from build123d import *

# Parameters (mm, degrees)
SKETCH1_W                              = 60
SKETCH1_H                              = 60
BOSS_EXTRUDE1_DEPTH                    = 3
SKETCH2_R                              = 10.25
CUT_EXTRUDE1_DEPTH                     = 43.532340636
SKETCH3_R                              = 1.45
SERVO_Y_MOUNT_D2P9_DEPTH               = 3.01
SKETCH4_R                              = 1.45
CUT_EXTRUDE5_DEPTH                     = 43.532340636
SKETCH5_R                              = 1.2
GUIDERAIL1_D2P4_DEPTH                  = 3.01
SKETCH6_R                              = 1.2
GUIDEBLOCK2_D2P4_DEPTH                 = 3.01
SKETCH7_R                              = 2.1
GUIDEBLOCK2_HEADCOUNTERBORE_D4P2_DEPTH = 2.05


with BuildPart() as part:
    # Sketch1 → Boss-Extrude1 (new body)
    with BuildSketch(Plane.XY):
        Rectangle(SKETCH1_W, SKETCH1_H)
    extrude(amount=BOSS_EXTRUDE1_DEPTH)

    # Sketch2 → Cut-Extrude1 (cut, through all)
    with BuildSketch(Plane.XY.offset(3)):
        Circle(SKETCH2_R)
    extrude(amount=-CUT_EXTRUDE1_DEPTH, mode=Mode.SUBTRACT)

    # Sketch3 → Servo_Y_Mount_D2p9 (cut)
    with BuildSketch(Plane(origin=(0, 0, 0), x_dir=(-1, 0, 0), z_dir=(0, 0, -1))):
        with Locations((18, -25)):
            Circle(SKETCH3_R)
        with Locations((25, -25)):
            Circle(SKETCH3_R)
    extrude(amount=-SERVO_Y_MOUNT_D2P9_DEPTH, mode=Mode.SUBTRACT)

    # Sketch4 → Cut-Extrude5 (cut, through all)
    with BuildSketch(Plane(origin=(0, 0, 0), x_dir=(-1, 0, 0), z_dir=(0, 0, -1))):
        with Locations((17, 27)):
            Circle(SKETCH4_R)
        with Locations((23, 27)):
            Circle(SKETCH4_R)
    extrude(amount=-CUT_EXTRUDE5_DEPTH, mode=Mode.SUBTRACT)

    # Sketch5 → GuideRail1_D2p4 (cut)
    with BuildSketch(Plane.XY.offset(3)):
        with Locations((-24, -15)):
            Circle(SKETCH5_R)
        with Locations((-24, 0)):
            Circle(SKETCH5_R)
        with Locations((-24, 15)):
            Circle(SKETCH5_R)
    extrude(amount=-GUIDERAIL1_D2P4_DEPTH, mode=Mode.SUBTRACT)

    # Sketch6 → GuideBlock2_D2p4 (cut)
    with BuildSketch(Plane.XY.offset(3)):
        with Locations((0, -28)):
            Circle(SKETCH6_R)
        with Locations((0, -20)):
            Circle(SKETCH6_R)
    extrude(amount=-GUIDEBLOCK2_D2P4_DEPTH, mode=Mode.SUBTRACT)

    # Sketch7 → GuideBlock2_HeadCounterbore_D4p2 (cut)
    with BuildSketch(Plane.XY.offset(3)):
        with Locations((0, -28)):
            Circle(SKETCH7_R)
        with Locations((0, -20)):
            Circle(SKETCH7_R)
    extrude(amount=-GUIDEBLOCK2_HEADCOUNTERBORE_D4P2_DEPTH, mode=Mode.SUBTRACT)


solid = part.part
Geometry: final body of the model. Coordinates: model frame, mm. A direction names the side the tool comes from. Give positions to 0.01 mm unless a question says otherwise; leave off trailing zeros. Order: outer loops, then holes, each group sorted by start corner. A loop starts at its lowest first (then second) coordinate and runs counter-clockwise, first axis right, second up. Notation, with made-up numbers: (-5, -22.5) - (15, -22.5) arc R30 cw to (15, 7.5) - close; hole circle Ø1 at (-6, 20). An arc over 180 degrees is marked (long way). Use CSV: the item, a comma, the result in double quotes.
1. Section query C-C (x = -7.5). Output: boundary loops of the cut face in (y, z), plus the area to 3 significant figures.
Answers below:
outline,"(-30, 0) - (-6.99, 0) - (-6.99, 3) - (-30, 3) - close; (6.99, 0) - (30, 0) - (30, 3) - (6.99, 3) - close"
area,"138 mm2"
2. Mould query, pull axis Y, two halves, no side actions, for faces 1 (the face through (30, 0, 1)), 2 (the face through (-0.4, -30, 0.8)), 3 (the face through (-19.339, -25.555, 1.479)). Classes: +Y half, -Y half, draft (parallel to the pull), parting line (faces both ways), or undercut.
Answers below:
face 1,"draft"
face 2,"-Y half"
face 3,"undercut"
3. Access query for faces 4 (the face through (1, -29, 0.95)), 5 (the face through (-25.2, 0.05, 1.52)). Directions: +Z, -Z, +X, -X, +Y, -Y. A direction counts if a zero-diameter tool reaches every point of the face in a straight line with its end or side. Return the directions, or none.
Answers below:
face 4,"+Z"
face 5,"+Z, -Z"
4. Contact query for a flat-ended pin moving along its axis: pin 1 (1.3 mm diameter, centred on x = 0.5, y = -21, fed in from +Z). Output: stop coordinate, or through.
Answers below:
pin 1,"z = 0.95"
5. Material intervals for line 1 along Y through (x, z) = (0, 2.3); line 2 along Y through (x, z) = (0, 0.4); line 3 along Y through (x, z) = (-24, 0.7), sorted ascending. Write a range as from..to.
Answers below:
line 1,"-25.9..-22.1, -17.9..-10.25, 10.25..30"
line 2,"-30..-29.2, -26.8..-21.2, -18.8..-10.25, 10.25..30"
line 3,"-30..-26.05, -23.95..-16.2, -13.8..-1.2, 1.2..13.8, 16.2..25.95, 28.05..30"
6. Section query D-D (y = 15). Output: boundary loops of the cut face in (x, z).
Answers below:
outline,"(-30, 0) - (-25.2, 0) - (-25.2, 3) - (-30, 3) - close; (-22.8, 0) - (30, 0) - (30, 3) - (-22.8, 3) - close"
7. Section query B-B (z = 2). Give the number of separate pieces and of enclosed holes in the cut face, plus the area to 3 significant figures.
Answers below:
separate pieces,"1"
enclosed holes,"9"
area,"3,200 mm2"
8. Section query A-A (y = -20). Output: boundary loops of the cut face in (x, z), plus the area to 3 significant figures.
Answers below:
outline,"(-30, 0) - (-1.2, 0) - (-1.2, 0.95) - (-2.1, 0.95) - (-2.1, 3) - (-30, 3) - close; (1.2, 0) - (30, 0) - (30, 3) - (2.1, 3) - (2.1, 0.95) - (1.2, 0.95) - close"
area,"169 mm2"
